Could you check a few things on this model? Use its own coordinates, in mm. A direction names the side the tool comes from. Give positions to 0.01 mm unless a question says otherwise; leave off trailing zeros. Write each loop counter-clockwise with the first axis right and the second up, starting at its lowest first coordinate (ties: lowest second). Pieces come first, ordered by that corner, then holes. Notation, with made-up numbers: (48, 48) - (103, 48) arc R11 cw to (103, 64) - close; hole circle Ø2 at (-25, -35.5). An arc over 180 degrees is marked (long way). Answer as CSV lines item,"result". Start each with the question number.
Q1. Imagine slicing it at D-D on x = 18.5. List the corners of the cut face in (y, z) for me.
Q2. On a 3-axis mill with a long thin cutter (end or side, diameter ignored), from which of +Z, -Z, +X, -X, +Y, -Y can I reach the whole of each face in a straight line? I mean faces 1 (the face through (-213, -41, -85.852)), 2 (the face through (-84, -4.762, -49)), 3 (the face through (-111, 58.674, -91)), 4 (the face through (-87, 41, -12.7)). Say none if no direction works.
Q3. Will these pins go through, and if not, where does the flat tip stop? pin 1 Ø1 at (x, y) = (20, -57) entering from +Z; pin 2 Ø8 at (y, z) = (-27, -122.5) entering from -X (3 decimals); pin 3 Ø12 at (y, z) = (50.8, -127.254) entering from +X; pin 4 Ø21 at (x, z) = (-199.5, -122) entering from -Y.
Q4. Imagine slicing it at B-B on y = -30.5. List the corners of the cut face in (x, z) for me (3 decimals).
Q5. Imagine slicing it at C-C on z = -41.5. List the corners of the cut face in (x, y) for me (1 decimal).
Q6. If I drill on line 1 along X through (y, z) = (29, -25.5) (3 decimals); line 2 along Y through (x, z) = (150, -90); line 3 along Z through (x, y) = (-188, 14), over which ranges is the centre line in solid material (lowest first)?
Q7. We'd pull the mould along Z, two halves only. Please class faces 5 (the face through (-196.72, 49.34, -133.84)), 6 (the face through (-106, -69.85, 5)): pulls with the +Z half, pulls with the -Z half, needs draft (parallel to the pull), parting line crosses it, or undercut.
Q8. Imagine slicing it at A-A on x = 166. State how many separate pieces and enclosed holes the cut face has, and give its area (3 significant figures).
```python
from build123d import *

# Parameters (mm, degrees)
F0_W      = 438.15
F0_H      = 152.4
F1_DEPTH  = 12.7
F2_W      = 152.4
F2_H      = 139.7
F3_DEPTH  = 9.525
F4_W      = 9.652
F4_H      = 71.4375
F4_H_2    = 9.525
F4_W_2    = 12.7
F4_W_3    = 222.25
F4_W_4    = 174.244
F5_DEPTH  = 73.152
F6_W      = 438.15
F6_H      = 152.4
F7_DEPTH  = 9.652
F9_DEPTH  = 25.4
F11_D     = 10.0838
F11_DEPTH = 38.1
F11_TIP   = 3.0294791551
F12_W     = 158.75
F12_H     = 152.4
F13_DEPTH = 3.175
F15_D     = 7.9375
F15_DEPTH = 38.1
F15_TIP   = 2.3846655818
F16_W     = 19.05
F16_H     = 127
F17_DEPTH = 50.8
F19_D     = 13.49248
F19_DEPTH = 21.2274727273
F19_TIP   = 4.0535499425


with BuildPart() as f1:
    # F0 (on Top) → F1 (new body)
    with BuildSketch(Plane.XY):
        Rectangle(F0_W, F0_H)
    extrude(amount=-F1_DEPTH)

    # F2 (on face) → F3 (join)
    with BuildSketch(Plane.XY):
        with Locations((-104.775, 0)):
            Rectangle(F2_W, F2_H)
    extrude(amount=F3_DEPTH)

    # F4 (on face) → F5 (join)
    with BuildSketch(Plane(origin=(0, 0, -12.7), x_dir=(1, 0, 0), z_dir=(0, 0, -1))):
        with Locations((-201.549, 40.48125)):
            Rectangle(F4_W, F4_H)
        with Locations((-201.549, 0)):
            Rectangle(F4_W, F4_H_2)
        with Locations((-212.725, 0)):
            Rectangle(F4_W_2, F4_H_2)
        with Locations((-85.598, 0)):
            Rectangle(F4_W_3, F4_H_2)
        with Locations((-201.549, -40.48125)):
            Rectangle(F4_W, F4_H)
        with Locations((30.353, 0)):
            Rectangle(F4_W, F4_H_2)
        with Locations((30.353, 40.48125)):
            Rectangle(F4_W, F4_H)
        with Locations((30.353, -40.48125)):
            Rectangle(F4_W, F4_H)
        with Locations((122.301, 0)):
            Rectangle(F4_W_4, F4_H_2)
        with Locations((214.249, 0)):
            Rectangle(F4_W, F4_H_2)
        with Locations((214.249, 40.48125)):
            Rectangle(F4_W, F4_H)
        with Locations((214.249, -40.48125)):
            Rectangle(F4_W, F4_H)
    extrude(amount=F5_DEPTH)

    # F6 (on face) → F7 (join)
    with BuildSketch(Plane(origin=(0, 0, -85.852), x_dir=(1, 0, 0), z_dir=(0, 0, -1))):
        Rectangle(F6_W, F6_H)
    extrude(amount=F7_DEPTH)

    # F8 (on face) → F9 (cut)
    with BuildSketch(Plane(origin=(0, 0, -95.504), x_dir=(1, 0, 0), z_dir=(0, 0, -1))):
        with BuildLine():
            Line((-130.175, 44.45), (-92.075, 44.45))
            ThreePointArc((-92.075, 44.45), (-84.963, 51.562), (-92.075, 58.674))
            Line((-92.075, 58.674), (-130.175, 58.674))
            ThreePointArc((-130.175, 58.674), (-137.287, 51.562), (-130.175, 44.45))
        make_face()
        with BuildLine():
            ThreePointArc((-130.175, -44.45), (-137.287, -51.562), (-130.175, -58.674))
            Line((-130.175, -58.674), (-92.075, -58.674))
            ThreePointArc((-92.075, -58.674), (-84.963, -51.562), (-92.075, -44.45))
            Line((-92.075, -44.45), (-130.175, -44.45))
        make_face()
        with BuildLine():
            Line((187.325, 58.674), (149.225, 58.674))
            ThreePointArc((149.225, 58.674), (142.113, 51.562), (149.225, 44.45))
            Line((149.225, 44.45), (187.325, 44.45))
            ThreePointArc((187.325, 44.45), (194.437, 51.562), (187.325, 58.674))
        make_face()
        with BuildLine():
            ThreePointArc((149.225, -44.45), (142.113, -51.562), (149.225, -58.674))
            Line((149.225, -58.674), (187.325, -58.674))
            ThreePointArc((187.325, -58.674), (194.437, -51.562), (187.325, -44.45))
            Line((187.325, -44.45), (149.225, -44.45))
        make_face()
    extrude(amount=-F9_DEPTH, mode=Mode.SUBTRACT)

    # F11
    with Locations(Plane.XY.offset(9.525)):
        with Locations((-156.337, 51.562), (-53.213, 51.562), (-156.337, -51.562), (-53.213, -51.562)):
            Hole(F11_D / 2, depth=F11_DEPTH)
            with Locations((0, 0, -(F11_DEPTH + F11_TIP / 2))):  # 118° drill point
                Cone(0, F11_D / 2, F11_TIP, mode=Mode.SUBTRACT)

    # F12 (on face) → F13 (cut)
    with BuildSketch(Plane.XY):
        with Locations((139.7, 0)):
            Rectangle(F12_W, F12_H)
    extrude(amount=-F13_DEPTH, mode=Mode.SUBTRACT)

    # F15
    with Locations(Plane.XY.offset(-3.175)):
        with Locations((106.299, 53.848), (176.149, 53.848), (176.149, -54.102), (106.299, -54.102)):
            Hole(F15_D / 2, depth=F15_DEPTH)
            with Locations((0, 0, -(F15_DEPTH + F15_TIP / 2))):  # 118° drill point
                Cone(0, F15_D / 2, F15_TIP, mode=Mode.SUBTRACT)

    # F16 (on face) → F17 (join)
    with BuildSketch(Plane(origin=(0, 0, -95.504), x_dir=(1, 0, 0), z_dir=(0, 0, -1))):
        with Locations((-196.85, 0)):
            Rectangle(F16_W, F16_H)
    extrude(amount=F17_DEPTH)

    # F19
    with Locations(Plane(origin=(-206.375, 0, 0), x_dir=(0, -1, 0), z_dir=(-1, 0, 0))):
        with Locations((50.8, -127.254), (-50.8, -127.254)):
            Hole(F19_D / 2, depth=F19_DEPTH)
            with Locations((0, 0, -(F19_DEPTH + F19_TIP / 2))):  # 118° drill point
                Cone(0, F19_D / 2, F19_TIP, mode=Mode.SUBTRACT)


solid = f1.part
```
Conclusion:
1,outline,"(-76.2, -95.5) - (76.2, -95.5) - (76.2, -85.85) - (4.76, -85.85) - (4.76, -12.7) - (76.2, -12.7) - (76.2, 0) - (-76.2, 0) - (-76.2, -12.7) - (-4.76, -12.7) - (-4.76, -85.85) - (-76.2, -85.85) - close"
2,face 1,"-X, -Y"
2,face 2,"-Y"
2,face 3,"-Z"
2,face 4,"+Y"
3,pin 1,"z = 0"
3,pin 2,"x = -206.375"
3,pin 3,"through"
3,pin 4,"y = -63.5"
4,outline,"(-219.075, -95.504) - (-206.375, -95.504) - (-206.375, -146.304) - (-187.325, -146.304) - (-187.325, -95.504) - (219.075, -95.504) - (219.075, -3.175) - (60.325, -3.175) - (60.325, 0) - (-28.575, 0) - (-28.575, 9.525) - (-180.975, 9.525) - (-180.975, 0) - (-219.075, 0) - (-219.075, -12.7) - (-206.375, -12.7) - (-206.375, -85.852) - (-219.075, -85.852) - close; hole (-196.723, -85.852) - (25.527, -85.852) - (25.527, -12.7) - (-196.723, -12.7) - close; hole (35.179, -85.852) - (209.423, -85.852) - (209.423, -12.7) - (35.179, -12.7) - close"
5,outline,"(-219.1, -4.8) - (-206.4, -4.8) - (-206.4, -76.2) - (-196.7, -76.2) - (-196.7, -4.8) - (25.5, -4.8) - (25.5, -76.2) - (35.2, -76.2) - (35.2, -4.8) - (209.4, -4.8) - (209.4, -76.2) - (219.1, -76.2) - (219.1, 76.2) - (209.4, 76.2) - (209.4, 4.8) - (35.2, 4.8) - (35.2, 76.2) - (25.5, 76.2) - (25.5, 4.8) - (-196.7, 4.8) - (-196.7, 76.2) - (-206.4, 76.2) - (-206.4, 4.8) - (-219.1, 4.8) - close"
6,line 1,"-206.375 to -196.723, 25.527 to 35.179, 209.423 to 219.075"
6,line 2,"-76.2 to -58.67, -44.45 to 44.45, 58.67 to 76.2"
6,line 3,"-146.3 to -85.85, -12.7 to 0"
7,face 5,"undercut"
7,face 6,"needs draft"
8,separate pieces,"3"
8,enclosed holes,"0"
8,area,"3,340 mm^2"
